The listing builds one solid part. Answer for the finished solid, in the listing's coordinates (mm). Face numbers are marked on the shaded views. A direction names the side the tool comes from. Coordinates: 2 decimals unless noted, no trailing zeros. Loops run counter-clockwise (first coordinate to the right, second up) from the corner with the lowest first, then second, coordinate; pieces in that order, holes last. Notation, with made-up numbers: (89.25, -2) - (142.25, -2) arc R15 ccw to (142.25, 14) - close; hole circle Ø11 at (74.25, 68). An arc over 180 degrees is marked (long way). Return JSON: item names as keys, results as strings. Group by question number.
1. Section C-C (z = 5.5) is taken. Write down the section's boundary in (x, y).
2. Section A-A (x = 0) is taken. Write down the section's boundary in (y, z), and give its area (3 significant figures).
3. Each of these flat-tipped pins is pushed along its axis until it touches: P1, Ø20, axis at y = -44, z = 14.5, coming from the +X side; P2, Ø4, axis at x = 11.5, z = 5, coming from the +Y side; P3, Ø8, axis at y = -2.5, z = 24.5, coming from the -X side. Where does it stop, or does it pass through?
4. Find the intervals of material crossed by line 1 along Y through (x, z) = (1, 19.5); line 2 along X through (y, z) = (-23, 31.5); line 3 along X through (y, z) = (-23.5, 2.5), in increasing order.
5. Section D-D (x = 23) is taken. Write down the section's boundary in (y, z), and give its area (3 significant figures).
6. The mould has two halves that part along X. Classify the marked faces 1, 2 and 3: pulls with the +X half, pulls with the -X half, needs draft (parallel to the pull), parting line crosses it, or undercut.
7. Which of the six approach directions +Z, -Z, +X, -X, +Y, -Y give full straight-line access (tool end or side, diameter ignored) to the marked faces 4, 5 and 6?
8. Section B-B (y = 0) is taken. Write down the section's boundary in (x, z), and give its area (3 significant figures).
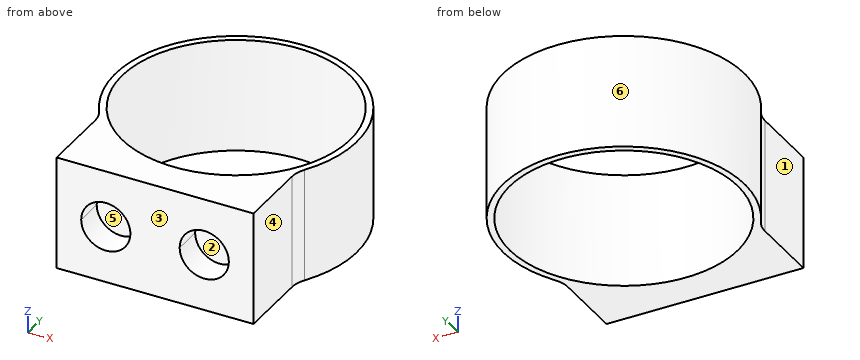
```python
from build123d import *

# Parameters (mm, degrees)
SKETCH1_R           = 40
BOSS_EXTRUDE1_DEPTH = 40
CUT_EXTRUDE2_DEPTH  = 10
FILLET1_R           = 10


with BuildPart() as part:
    # Sketch1 → Boss-Extrude1 (new body)
    with BuildSketch(Plane.XY):
        with BuildLine():
            Line((-34.599296367, -24.44828034), (-34.599296367, -52.365409812))
            Line((-34.599296367, -52.365409812), (34.599296367, -52.365409812))
            Line((34.599296367, -52.365409812), (34.599296367, -24.44828034))
            ThreePointArc((34.599296367, -24.44828034), (0, 42.365430727), (-34.599296367, -24.44828034))
        make_face()
        Circle(SKETCH1_R, mode=Mode.SUBTRACT)
    extrude(amount=BOSS_EXTRUDE1_DEPTH)

    # Sketch4 → Cut-Extrude2 (cut)
    with BuildSketch(Plane(origin=(0, -52.365409812, 0), x_dir=(-1, 0, 0), z_dir=(0, -1, 0))):
        with BuildLine():
            ThreePointArc((8.655703751, -20), (17.299648183, -28.643944432), (25.943592616, -20))
            Line((25.943592616, -20), (8.655703751, -20))
        make_face()
        with BuildLine():
            Line((8.655703751, -20), (25.943592616, -20))
            ThreePointArc((25.943592616, -20), (17.299648183, -11.356055568), (8.655703751, -20))
        make_face()
        with BuildLine():
            ThreePointArc((-25.943592616, -20), (-17.299648183, -28.643944432), (-8.655703751, -20))
            Line((-8.655703751, -20), (-25.943592616, -20))
        make_face()
        with BuildLine():
            Line((-25.943592616, -20), (-8.655703751, -20))
            ThreePointArc((-8.655703751, -20), (-17.299648183, -11.356055568), (-25.943592616, -20))
        make_face()
    extrude(amount=-CUT_EXTRUDE2_DEPTH, mode=Mode.SUBTRACT)

    # Fillet1
    fillet1_edges = [part.edges().sort_by_distance(p)[0] for p in [
        (-34.599296367, -24.44828034, 20),
        (34.599296367, -24.44828034, 20),
    ]]
    fillet(fillet1_edges, radius=FILLET1_R)


solid = part.part
```
The answers:
{
 "1": {"outline": "(-36.08, -22.2) arc R10 cw to (-34.6, -27.44) - (-34.6, -52.37) - (34.6, -52.37) - (34.6, -27.44) arc R10 cw to (36.08, -22.2) arc R42.37 ccw (long way) to start; hole circle Ø80 at (0, 0)"},
 "2": {"outline": "(-52.37, 0) - (-40, 0) - (-40, 40) - (-52.37, 40) - close; (40, 0) - (42.37, 0) - (42.37, 40) - (40, 40) - close", "area": "589 mm2"},
 "3": {"P1": "stops at x = 34.6", "P2": "stops at y = 41.29", "P3": "stops at x = -42.37"},
 "4": {"line 1": "y = -52.37 to -39.99, 39.99 to 42.35", "line 2": "x = -35.64 to -32.73, 32.73 to 35.64", "line 3": "x = -35.41 to -32.37, 32.37 to 35.41"},
 "5": {"outline": "(-52.37, 0) - (-32.73, 0) - (-32.73, 40) - (-52.37, 40) - (-52.37, 26.5) - (-42.37, 26.5) - (-42.37, 13.5) - (-52.37, 13.5) - close; (32.73, 0) - (35.58, 0) - (35.58, 40) - (32.73, 40) - close", "area": "770 mm2"},
 "6": {"face 1": "pulls with the -X half", "face 2": "undercut", "face 3": "needs draft"},
 "7": {"face 4": "+Z, -Z, +X, -Y", "face 5": "-Y", "face 6": "+Z, -Z"},
 "8": {"outline": "(-42.37, 0) - (-40, 0) - (-40, 40) - (-42.37, 40) - close; (40, 0) - (42.37, 0) - (42.37, 40) - (40, 40) - close", "area": "189 mm2"}
}
